Design review of the part built by this model. Coordinates are the model's own, in mm. A direction names the side the tool comes from. Give positions to 0.01 mm unless a question says otherwise; leave off trailing zeros. Loops run counter-clockwise (first coordinate to the right, second up) from the corner with the lowest first, then second, coordinate; pieces in that order, holes last. Notation, with made-up numbers: (-4.5, 15.25) - (28.5, 15.25) arc R22 ccw to (28.5, 54.25) - close; hole circle Ø5 at (62.5, 9.25). An arc over 180 degrees is marked (long way). Write each question's results on one line, items separated by ' | '.
```python
from build123d import *

# Parameters (mm, degrees)
SKETCH_1_W          = 48
SKETCH_1_H          = 43
EXTRUDE_1_DEPTH     = 5
SKETCH_2_W          = 32
SKETCH_2_H          = 40
CUT_EXTRUDE_1_DEPTH = 2.25
SKETCH_3_R          = 2.1
CUT_EXTRUDE_2_DEPTH = 65.637450445
CHAMFER_1_SIZE      = 2
FILLET_1_R          = 2
CHAMFER_2_SIZE      = 2
SKETCH_4_W          = 32
SKETCH_4_H          = 8.9
CUT_EXTRUDE_3_DEPTH = 65.502422435


with BuildPart() as part:
    # Эскиз1 → Бобышка-Вытянуть1 (new body)
    with BuildSketch(Plane(origin=(0, 0, 0), x_dir=(1, 0, 0), z_dir=(0, 1, 0))):
        with Locations((-24, 21.5)):
            Rectangle(SKETCH_1_W, SKETCH_1_H)
    extrude(amount=-EXTRUDE_1_DEPTH)

    # Эскиз2 → Вырез-Вытянуть1 (cut)
    with BuildSketch(Plane(origin=(0, 0, 0), x_dir=(1, 0, 0), z_dir=(0, 1, 0))):
        with Locations((-24, 20)):
            Rectangle(SKETCH_2_W, SKETCH_2_H)
    extrude(amount=-CUT_EXTRUDE_1_DEPTH, mode=Mode.SUBTRACT)

    # Эскиз3 → Вырез-Вытянуть2 (cut, through all)
    with BuildSketch(Plane(origin=(0, 0, 0), x_dir=(1, 0, 0), z_dir=(0, 1, 0))):
        with Locations(Location((-44, 39, 0), (0, 0, 270))):
            Circle(SKETCH_3_R)
        with Locations(Location((-4, 39, 0), (0, 0, 90))):
            Circle(SKETCH_3_R)
        with Locations(Location((-4, 4, 0), (0, 0, 270))):
            Circle(SKETCH_3_R)
        with Locations(Location((-44, 4, 0), (0, 0, 90))):
            Circle(SKETCH_3_R)
    extrude(amount=-CUT_EXTRUDE_2_DEPTH, mode=Mode.SUBTRACT)

    # Фаска1
    # the kernel refuses this chamfer: 2 mm, written as the material it takes off along each edge
    with BuildSketch(Plane(origin=(-44, -5, -4), x_dir=(0, 0, -1), z_dir=(1, 0, 0))) as chamfer_1_piece_1:
        Polygon((2.1 + CHAMFER_1_SIZE, 0), (2.1, CHAMFER_1_SIZE), (2.1, 0), align=None)
    revolve(axis=Axis((-44, -5, -4), (0, 1, 0)), mode=Mode.SUBTRACT)
    with BuildSketch(Plane(origin=(-4, -5, -4), x_dir=(0, 0, 1), z_dir=(-1, 0, 0))) as chamfer_1_piece_2:
        Polygon((2.1 + CHAMFER_1_SIZE, 0), (2.1, CHAMFER_1_SIZE), (2.1, 0), align=None)
    revolve(axis=Axis((-4, -5, -4), (0, 1, 0)), mode=Mode.SUBTRACT)
    with BuildSketch(Plane(origin=(-4, -5, -39), x_dir=(0, 0, -1), z_dir=(1, 0, 0))) as chamfer_1_piece_3:
        Polygon((2.1 + CHAMFER_1_SIZE, 0), (2.1, CHAMFER_1_SIZE), (2.1, 0), align=None)
    revolve(axis=Axis((-4, -5, -39), (0, 1, 0)), mode=Mode.SUBTRACT)
    with BuildSketch(Plane(origin=(-44, -5, -39), x_dir=(0, 0, 1), z_dir=(-1, 0, 0))) as chamfer_1_piece_4:
        Polygon((2.1 + CHAMFER_1_SIZE, 0), (2.1, CHAMFER_1_SIZE), (2.1, 0), align=None)
    revolve(axis=Axis((-44, -5, -39), (0, 1, 0)), mode=Mode.SUBTRACT)

    # Скругление1
    fillet_1_edges = [part.edges().sort_by_distance(p)[0] for p in [
        (-48, -2.5, -43),
        (0, -2.5, -43),
        (0, -2.5, 0),
        (-48, -2.5, 0),
    ]]
    fillet(fillet_1_edges, radius=FILLET_1_R)

    # Фаска2
    chamfer_2_edges = [part.edges().sort_by_distance(p)[0] for p in [
        (-24, 0, -40),
    ]]
    chamfer(chamfer_2_edges, length=CHAMFER_2_SIZE)

    # Эскиз4 → Вырез-Вытянуть3 (cut, through all)
    with BuildSketch(Plane(origin=(0, -2.25, 0), x_dir=(1, 0, 0), z_dir=(0, 1, 0))):
        with Locations((-24, 4.45)):
            Rectangle(SKETCH_4_W, SKETCH_4_H)
    extrude(amount=-CUT_EXTRUDE_3_DEPTH, mode=Mode.SUBTRACT)


solid = part.part
```
Item 1: Wall thickness on probe 1 along X at (y, z) = (-1.95, -4); probe 2 along X at (y, z) = (-1.15, -13.5); probe 3 along X at (y, z) = (-1.9, -3): over which ranges is each line inside the solid? List them lowest first.
Output values:
probe 1: x = -48 to -46.1, -41.9 to -40, -8 to -6.1, -1.9 to 0 | probe 2: x = -48 to -40, -8 to 0 | probe 3: x = -48 to -45.85, -42.15 to -40, -8 to -5.85, -2.15 to 0
Item 2: We need section D-D on z = -39. Give the boundary of the cut face in (x, y).
Output values:
outline: (-48, -4.9) - (-46.1, -3) - (-46.1, 0) - (-48, 0) - close; (-41.9, -3) - (-39.9, -5) - (-8.1, -5) - (-6.1, -3) - (-6.1, 0) - (-8, 0) - (-8, -2.25) - (-40, -2.25) - (-40, 0) - (-41.9, 0) - close; (-1.9, -3) - (0, -4.9) - (0, 0) - (-1.9, 0) - close
Item 3: Draft analysis for pull direction Z (two halves, no side actions). For faces 4 (the face through (-8, -1, -16)), 5 (the face through (-24, -1, -41)), 6 (the face through (-6.05, -1.48, -4.46)), 7 (the face through (-42.137, -1.479, -4.969)), state which applies: +Z half, -Z half, draft (parallel to the pull), parting line (faces both ways), or undercut.
Output values:
face 4: draft | face 5: +Z half | face 6: undercut | face 7: undercut
Item 4: Clearance check with flat-ended pins moving along their axes: P1, Ø4, axis at x = -4, z = -39, coming from the -Y side; P2, Ø3, axis at x = -25, y = -4, coming from the +Z side; P3, Ø15.5, axis at x = -26.5, z = -22, coming from the +Y side; P4, Ø6.5, axis at x = -44, z = -4, coming from the +Y side. State where each tip first meets the part, or that it passes through.
Output values:
P1: passes through | P2: stops at z = -8.9 | P3: stops at y = -2.25 | P4: stops at y = 0
Item 5: We need section A-A on y = -4.05. Give the boundary of the cut face in (x, z), then the cut area to 3 significant figures.
Output values:
outline: (-48, -41) arc R2 ccw to (-46, -43) - (-2, -43) arc R2 ccw to (0, -41) - (0, -2) arc R2 ccw to (-2, 0) - (-8, 0) - (-8, -8.9) - (-40, -8.9) - (-40, 0) - (-46, 0) arc R2 ccw to (-48, -2) - close; hole circle Ø6.3 at (-44, -39); hole circle Ø6.3 at (-44, -4); hole circle Ø6.3 at (-4, -39); hole circle Ø6.3 at (-4, -4) | area: 1,650 mm²
Item 6: We need section C-C on x = -4. Give the boundary of the cut face in (y, z), then the cut area to 3 significant figures.
Output values:
outline: (-5, -34.9) - (-3, -36.9) - (0, -36.9) - (0, -6.1) - (-3, -6.1) - (-5, -8.1) - close; (-4.9, -43) - (0, -43) - (0, -41.1) - (-3, -41.1) - close; (-4.9, 0) - (-3, -1.9) - (0, -1.9) - (0, 0) - close | area: 165 mm²
Item 7: We need section B-B on z = -4. Give the boundary of the cut face in (x, y), then the cut area to 3 significant figures.
Output values:
outline: (-48, -4.9) - (-46.1, -3) - (-46.1, 0) - (-48, 0) - close; (-41.9, -3) - (-40, -4.9) - (-40, 0) - (-41.9, 0) - close; (-8, -4.9) - (-6.1, -3) - (-6.1, 0) - (-8, 0) - close; (-1.9, -3) - (0, -4.9) - (0, 0) - (-1.9, 0) - close | area: 30.0 mm²
Item 8: Tool access review of faces 1 (the face through (0, -2, -21)), 2 (the face through (-40, -1, -16)), 3 (the face through (-24, -4, -8.9)): name each direction out of +Z, -Z, +X, -X, +Y, -Y from which nothing blocks a thin tool from reaching the whole face with its end or side.
Output values:
face 1: +Z, -Z, +X, +Y, -Y | face 2: +Z, +Y | face 3: +Z, +Y, -Y
